Check sheet for the modelled part. Datum: model origin and axes. Units: mm. A direction names the side the tool comes from. Give positions to 0.01 mm unless a question says otherwise; leave off trailing zeros. Write each loop counter-clockwise with the first axis right and the second up, starting at its lowest first coordinate (ties: lowest second). Pieces come first, ordered by that corner, then holes. Notation, with made-up numbers: M 12,75.5 L 48,75.5 A36 ccw 48,111.5 Z; hole C 38.5,-6 d2. An arc over 180 degrees is marked long. Write item = value, one per line. Start each with the question number.
1) Sectioned sample at A-A, the plane x = -31.5. Record the cut outline in (y, z).
2) Draft check along Y on faces 1 (the face through (-12, 1.524, -33)), 2 (the face through (-12, 0, -33)), 3 (the face through (10.195, 1, -6)). Enter one of: pulls with the +Y half, pulls with the -Y half, needs draft (parallel to the pull), parting line crosses it, or undercut.
3) Sectioned sample at B-B, the plane z = -23. Record the cut outline in (x, y), then the cut area to 3 significant figures.
4) Gauge pin test, flat ends, axial feed: pin 1 (0.8 mm diameter, centred on x = -38, y = 0.5, fed in from +Z); pin 2 (12 mm diameter, centred on x = -25.5, z = -29.5, fed in from -Y); pin 3 (0.5 mm diameter, centred on y = 0.5, z = -51.5, fed in from -X); pin 4 (0.5 mm diameter, centred on y = 1, z = -5.5, fed in from +X). Record the tip position at first contact, or that the pin passes through.
5) Sectioned sample at C-C, the plane y = 1.05. Count the separate pieces of the cut face and the enclosed holes in it, then the cut area to 3 significant figures.
6) Scan lines: L1, parallel to Z at x = 7, y = 1.35; L2, parallel to Z at x = -9, y = 0.35; L3, parallel to X at y = 0.25, z = -43.5. Record each from-to range of solid material in increasing order.
7) Set-up check for faces 4 (the face through (-29.683, 1, -14)), 5 (the face through (10.195, 1, -51)), 6 (the face through (13, 1, -8.734)): record each of +Z, -Z, +X, -X, +Y, -Y from which the full face is reachable in a straight line by a thin tool's end or side.
Autodesk Inventor part; units mm, degrees
ref_plane "YZ Plane" through (0, 0, 0) normal (1, 0, 0) x (0, 1, 0)
ref_plane "XZ Plane" through (0, 0, 0) normal (0, 1, 0) x (-1, 0, 0)
ref_plane "XY Plane" through (0, 0, 0) normal (0, 0, 1) x (1, 0, 0)
sketch "Sketch1" plane through (0, 0, 0) normal (0, 1, 0) x (-1, 0, 0)
  line L0 (38.3189, -53.1839) -> (-10.1951, -53.1839)
  line L1 (-10.1951, -53.1839) -> (-10.1951, -49.0183)
  line L2 (-10.1951, -49.0183) -> (-16.5451, -49.0183)
  line L3 (-16.5451, -49.0183) -> (-16.5451, -8.7339)
  line L4 (-16.5451, -8.7339) -> (-10.1951, -8.7339)
  line L5 (-10.1951, -8.7339) -> (-10.1951, -2.3839)
  line L6 (-10.1951, -2.3839) -> (29.6829, -2.3839)
  line L7 (29.6829, -2.3839) -> (29.6829, -25.4471)
  line L8 (29.6829, -25.4471) -> (40.6049, -25.4471)
  line L9 (40.6049, -25.4471) -> (40.6049, -49.0183)
  line L10 (40.6049, -49.0183) -> (38.3189, -49.0183)
  line L11 (38.3189, -49.0183) -> (38.3189, -53.1839)
  circle A0 centre (37.8363, -43.6589) radius 0.4445
  circle A1 centre (35.2963, -43.6589) radius 0.4445
  circle A2 centre (37.6077, -28.1395) radius 0.4445
  circle A3 centre (35.0677, -28.1395) radius 0.4445
  circle A4 centre (19.1165, -44.7765) radius 0.4445
  circle A5 centre (16.5765, -44.7765) radius 0.4445
  circle A6 centre (14.0365, -44.7765) radius 0.4445
  circle A7 centre (11.4965, -44.7765) radius 0.4445
  circle A8 centre (8.9565, -44.7765) radius 0.4445
  circle A9 centre (6.4165, -44.7765) radius 0.4445
  circle A10 centre (3.8765, -44.7765) radius 0.4445
  circle A11 centre (1.3365, -44.7765) radius 0.4445
  circle A12 centre (19.1165, -26.9965) radius 0.4445
  circle A13 centre (16.5765, -26.9965) radius 0.4445
  circle A14 centre (14.0365, -26.9965) radius 0.4445
  circle A15 centre (11.4965, -26.9965) radius 0.4445
  circle A16 centre (8.9565, -26.9965) radius 0.4445
  circle A17 centre (6.4165, -26.9965) radius 0.4445
  circle A18 centre (3.8765, -26.9965) radius 0.4445
  circle A19 centre (1.3365, -26.9965) radius 0.4445
  circle A20 centre (19.1165, -20.6465) radius 0.4445
  circle A21 centre (16.5765, -20.6465) radius 0.4445
  circle A22 centre (14.0365, -20.6465) radius 0.4445
  circle A23 centre (11.4965, -20.6465) radius 0.4445
  circle A24 centre (8.9565, -20.6465) radius 0.4445
  circle A25 centre (6.4165, -20.6465) radius 0.4445
  circle A26 centre (3.8765, -20.6465) radius 0.4445
  circle A27 centre (18.9387, -32.5591) radius 0.4445
  circle A28 centre (16.3987, -32.5591) radius 0.4445
  circle A29 centre (13.8587, -32.5591) radius 0.4445
  circle A30 centre (11.3187, -32.5591) radius 0.4445
  circle A31 centre (-6.9439, -4.6953) radius 0.4445
  circle A32 centre (-6.9439, -7.2353) radius 0.4445
  circle A33 centre (-6.9439, -9.7753) radius 0.4445
  circle A34 centre (-6.9439, -12.3153) radius 0.4445
  circle A35 centre (-4.9119, -31.5939) radius 0.4445
  circle A36 centre (-4.9119, -34.1339) radius 0.4445
  point P0 (0, 0)
  dimension "d0" = 57.15
  dimension "d1" = 50.8
  dimension "d2" = 4.1656
  dimension "d3" = 6.35
  dimension "d4" = 6.35
  dimension "d5" = 10.922
  dimension "d6" = 23.0632
  dimension "d7" = 2.286
  dimension "d8" = 0.889
  dimension "d9" = 2.54
  dimension "d10" = 2.7686
  dimension "d11" = 9.525
  dimension "d12" = 0.889
  dimension "d13" = 2.54
  dimension "d14" = 2.6924
  dimension "d15" = 2.9972
  dimension "d16" = 2.54
  dimension "d17" = 2.54
  dimension "d18" = 2.54
  dimension "d19" = 2.54
  dimension "d20" = 2.54
  dimension "d21" = 2.54
  dimension "d22" = 2.54
  dimension "d23" = 8.4074
  dimension "d24" = 21.4884
  dimension "d25" = 2.54
  dimension "d26" = 2.54
  dimension "d27" = 2.54
  dimension "d28" = 2.54
  dimension "d29" = 2.54
  dimension "d30" = 2.54
  dimension "d31" = 2.54
  dimension "d32" = 17.78
  dimension "d33" = 2.54
  dimension "d34" = 2.54
  dimension "d35" = 2.54
  dimension "d36" = 2.54
  dimension "d37" = 2.54
  dimension "d38" = 2.54
  dimension "d39" = 6.35
  dimension "d40" = 2.54
  dimension "d41" = 2.54
  dimension "d42" = 2.54
  dimension "d44" = 2.54
  dimension "d45" = 2.54
  dimension "d46" = 2.54
  dimension "d47" = 2.3114
  dimension "d48" = 3.2512
  dimension "d49" = 0.1778
  dimension "d50" = 5.5626
  dimension "d51" = 2.54
  dimension "d52" = 14.8844
  dimension "d53" = 11.6332
extrude "Extrusion1" add sketch "Sketch1" along normal blind 1.524
properties part number "Main PCB2"
Data:
q1.outline = M 0,-53.18 L 1.52,-53.18 L 1.52,-25.45 L 0,-25.45 Z
q2.face_1 = pulls with the +Y half
q2.face_2 = pulls with the -Y half
q2.face_3 = needs draft
q3.outline = M -29.68,0 L 16.55,0 L 16.55,1.52 L -29.68,1.52 Z
q3.area = 70.5 mm2
q4.pin_1 = -25.45
q4.pin_2 = 0
q4.pin_3 = -38.32
q4.pin_4 = 10.2
q5.separate_pieces = 1
q5.enclosed_holes = 37
q5.area = 2,550 mm2
q6.L1 = -53.18 to -12.76, -11.87 to -10.22, -9.33 to -7.68, -6.79 to -5.14, -4.25 to -2.38
q6.L2 = -53.18 to -45.22, -44.33 to -27.44, -26.55 to -21.09, -20.2 to -2.38
q6.L3 = -40.6 to -38.25, -37.42 to -35.71, -34.88 to 16.55
q7.face_4 = +Z, -X, +Y, -Y
q7.face_5 = -Z, +X, +Y, -Y
q7.face_6 = +Z, +X, +Y, -Y
